The model under review builds one solid part; all positions refer to its coordinate system, in mm. Face numbers are marked on the shaded views. A direction names the side the tool comes from. Give positions to 0.01 mm unless a question says otherwise; leave off trailing zeros.
```python
from build123d import *

# Parameters (mm, degrees)
HEXAGONSOCKET_DEPTH = 1.1
HEADFILLET_R        = 0.1
CHAMFER_2_SIZE      = 0.2705
SKETCH4_W           = 5
SKETCH4_H           = 5
LPATTERN10_COUNT    = 18
LPATTERN10_PITCH    = 0.3246


with BuildPart() as part:
    # Sketch1 → Base (revolve)
    with BuildSketch(Plane.XY):
        Polygon((0, 0), (0, 3.36), (1.86, 1.5), (8, 1.5), (8, 0), align=None)
    revolve(axis=Axis((-0.587069181, 0, 0), (1, 0, 0)))

    # Sketch2 → HexagonSocket (cut)
    with BuildSketch(Plane(origin=(0, 0, 0), x_dir=(0, 0, -1), z_dir=(1, 0, 0))):
        Polygon((1.154700538, 0), (0.577350269, 1), (-0.577350269, 1), (-1.154700538, 0), (-0.577350269, -1), (0.577350269, -1), align=None)
    extrude(amount=HEXAGONSOCKET_DEPTH, mode=Mode.SUBTRACT)

    # Sketch3 → Cut-Revolve1 (revolve, cut)
    with BuildSketch(Plane.XY):
        Polygon((1.1, 1), (1.677350269, 0), (1.1, 0), align=None)
    revolve(axis=Axis((-0.439109555, 0, 0), (1, 0, 0)), mode=Mode.SUBTRACT)

    # HeadFillet
    headfillet_edges = [part.edges().sort_by_distance(p)[0] for p in [
        (1.86, -1.5, 0),
    ]]
    fillet(headfillet_edges, radius=HEADFILLET_R)

    # Chamfer 2
    chamfer_2_edges = [part.edges().sort_by_distance(p)[0] for p in [
        (8, -1.5, 0),
    ]]
    chamfer(chamfer_2_edges, length=CHAMFER_2_SIZE)

    # Sketch4 → Cut-Revolve2 (revolve, cut)
    with BuildSketch(Plane(origin=(0, 0, 0), x_dir=(1, 0, 0), z_dir=(0, 1, 0))):
        with Locations((0.5, 5.27)):
            Rectangle(SKETCH4_W, SKETCH4_H)
    revolve(axis=Axis((11.853138686, 0, 0), (-1, 0, 0)), mode=Mode.SUBTRACT)

    # Sketch5 → Cut-Revolve10 (revolve, cut)
    with BuildSketch(Plane.XY):
        Polygon((7.7295, 1.265740128), (7.86475, 1.5), (7.86475, 1.7705), (7.59425, 1.7705), (7.59425, 1.5), align=None)
    cut_revolve10 = revolve(axis=Axis((0, 0, 0), (1, 0, 0)), mode=Mode.SUBTRACT)

    # LPattern10: Cut-Revolve10 ×18
    with Locations(*[(-i * LPATTERN10_PITCH, 0, 0) for i in range(1, LPATTERN10_COUNT)]):
        add(cut_revolve10, mode=Mode.SUBTRACT)


solid = part.part
```
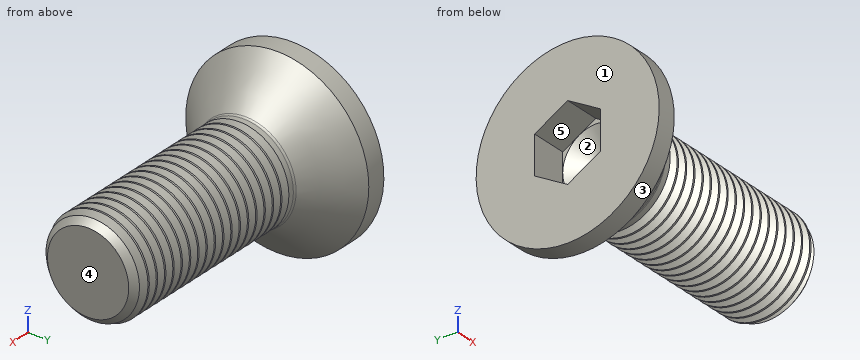
Item 1: For the marked faces 4 and 5, list the 3-axis set-ups (+Z, -Z, +X, -X, +Y, -Y) from which the entire face can be reached by the end or side of a thin tool; tool diameter is ignored.
Values found:
face 4: +Z, -Z, +X, +Y, -Y
face 5: -X
Item 2: For line 1 (X direction, y = 0.2, z = -2); line 2 (Y direction, x = 2, z = 1.05); line 3 (X direction, y = 1.75, z = 0.9), list the stretches that pass through material, from the lowest coordinate up.
Values found:
line 1: x = 0 to 1.35
line 2: y = -1.07 to 1.07
line 3: x = 0 to 1.39
Item 3: Draft analysis for pull direction Z (two halves, no side actions). For the marked faces 1, 2 and 3, state which applies: released by +Z, released by -Z, zero draft, split by the parting line, or undercut.
Values found:
face 1: zero draft
face 2: undercut
face 3: split by the parting line
Item 4: Clearance check with flat-ended pins moving along their axes: pin 1 Ø1.5 at (x, y) = (5, -2) entering from -Z; pin 2 Ø0.6 at (y, z) = (0.5, 0) entering from -X; pin 3 Ø1.5 at (x, z) = (3.5, 2) entering from +Y. State where each tip first meets the part, or that it passes through.
Values found:
pin 1: stops at z = -0.83
pin 2: stops at x = 1.22
pin 3: stops at y = 0.81
